from build123d import *

# Parameters (mm, degrees)
F0_R          = 25
F0_R_2        = 11.5
F1_DEPTH      = 17.5
F1_DEPTH_BACK = 17.5
F0_R_3        = 7.35
F2_DEPTH      = 6
F3_DEPTH      = 6
F4_R          = 8.4
F2_FACE_R     = 11.5
F2_FACE_R_2   = 7.35
F6_DEPTH      = 5
F3_FACE_R     = 11.5
F3_FACE_R_2   = 7.35
F7_DEPTH      = 3


with BuildPart() as f1:
    # F0 (on Front) → F1 (new body, two sides)
    with BuildSketch(Plane.XZ) as f1_sk:
        Circle(F0_R)
        Circle(F0_R_2, mode=Mode.SUBTRACT)
    extrude(amount=F1_DEPTH)
    extrude(f1_sk.sketch, amount=-F1_DEPTH_BACK)

    # F0 (on Front) → F2 (join)
    with BuildSketch(Plane.XZ):
        Circle(F0_R_2)
        Circle(F0_R_3, mode=Mode.SUBTRACT)
    extrude(amount=F2_DEPTH)

    # F0 (on Front) → F3 (join)
    with BuildSketch(Plane.XZ):
        Circle(F0_R_2)
        Circle(F0_R_3, mode=Mode.SUBTRACT)
    extrude(amount=-F3_DEPTH)

    # F4
    f4_edges = [f1.edges().sort_by_distance(p)[0] for p in [
        (-25, -17.5, 0),
        (-25, 17.5, 0),
    ]]
    fillet(f4_edges, radius=F4_R)

    # F2_face (on face) → F6 (cut)
    with BuildSketch(Plane.XZ.offset(6)):
        Circle(F2_FACE_R)
        Circle(F2_FACE_R_2, mode=Mode.SUBTRACT)
    extrude(amount=-F6_DEPTH, mode=Mode.SUBTRACT)

    # F3_face (on face) → F7 (join)
    with BuildSketch(Plane(origin=(0, 6, 0), x_dir=(1, 0, 0), z_dir=(0, 1, 0))):
        Circle(F3_FACE_R)
        Circle(F3_FACE_R_2, mode=Mode.SUBTRACT)
    extrude(amount=F7_DEPTH)


solid = f1.part
Here's how the part is built. I have some questions about the finished solid (model axes, mm). A direction names the side the tool comes from. Round coordinates to 2 decimals unless told otherwise and drop trailing zeros. Order: outer loops, then holes, each group sorted by start corner. A loop starts at its lowest first (then second) coordinate and runs counter-clockwise, first axis right, second up. Notation, with made-up numbers: M 49.25,14.25 L 88.25,14.25 A26 ccw 88.25,44.25 Z; hole C 83.5,18.25 d4. An arc over 180 degrees is marked long. Return JSON: item names as keys, results as strings. Group by question number.
1. I'm going to push flat-ended pins straight in: pin 1 Ø6 at (x, z) = (11.5, -18.5) entering from +Y; pin 2 Ø23.5 at (x, z) = (0, 0) entering from +Y; pin 3 Ø10 at (x, z) = (20, 11.5) entering from -Y; pin 4 Ø12 at (y, z) = (-3, 15) entering from +X. Where does each tip first touch, or does it pass through?
2. If we section it at B-B on z = 0: List the corners of the cut face in (x, y) for me.
3. Please list where these lines run through material, in increasing order: probe 1 along X at (y, z) = (-4, -0.5) (3 decimals); probe 2 along Z at (x, y) = (0, 0.75); probe 3 along Z at (x, y) = (0, -8).
4. If we section it at C-C on y = 1: List the corners of the cut face in (x, z) for me, then the cut area to 3 significant figures.
5. On a 3-axis mill with a long thin cutter (end or side, diameter ignored), from which of +Z, -Z, +X, -X, +Y, -Y can I reach the whole of each face in a straight line? I mean faces 5 (the face through (-4, 17.5, -11)), 6 (the face through (0, -1, -8)), 7 (the face through (-1.5, 13.2, 11.4)). Say none if no direction works.
6. If we mould it in two halves opening along Z, with no side actions, what happens to faces 1 (the face through (0, 9, 8)), 2 (the face through (-1.5, -9.1, 11.4)), 3 (the face through (23.846, -0.127, 7.509)), 4 (the face through (-4, -17.5, -11))? For each: pulls with the +Z half, pulls with the -Z half, needs draft (parallel to the pull), parting line crosses it, or undercut.
7. If we section it at A-A on x = 0: List the corners of the cut face in (y, z) for me.
8. If we section it at D-D on y = -7.5: List the corners of the cut face in (x, z) for me, then the cut area to 3 significant figures.
Reply:
{
 "1": {"pin 1": "y = 17.21", "pin 2": "y = 17.5", "pin 3": "y = -17.37", "pin 4": "x = 23.32"},
 "2": {"outline": "M -25,-9.1 A8.4 ccw -16.6,-17.5 L -11.5,-17.5 L -11.5,-1 L -7.35,-1 L -7.35,9 L -11.5,9 L -11.5,17.5 L -16.6,17.5 A8.4 ccw -25,9.1 Z; M 7.35,-1 L 11.5,-1 L 11.5,-17.5 L 16.6,-17.5 A8.4 ccw 25,-9.1 L 25,9.1 A8.4 ccw 16.6,17.5 L 11.5,17.5 L 11.5,9 L 7.35,9 Z"},
 "3": {"probe 1": "-24.995 to -11.489, 11.489 to 24.995", "probe 2": "-25 to -7.35, 7.35 to 25", "probe 3": "-25 to -11.5, 11.5 to 25"},
 "4": {"outline": "C 0,0 d50; hole C 0,0 d14.7", "area": "1,790 mm^2"},
 "5": {"face 5": "+Z, -Z, +X, -X, +Y", "face 6": "-Y", "face 7": "+Y"},
 "6": {"face 1": "undercut", "face 2": "undercut", "face 3": "parting line crosses it", "face 4": "needs draft"},
 "7": {"outline": "M -17.5,-16.6 A8.4 ccw -9.1,-25 L 9.1,-25 A8.4 ccw 17.5,-16.6 L 17.5,-11.5 L 9,-11.5 L 9,-7.35 L -1,-7.35 L -1,-11.5 L -17.5,-11.5 Z; M -17.5,11.5 L -1,11.5 L -1,7.35 L 9,7.35 L 9,11.5 L 17.5,11.5 L 17.5,16.6 A8.4 ccw 9.1,25 L -9.1,25 A8.4 ccw -17.5,16.6 Z"},
 "8": {"outline": "C 0,0 d50; hole C 0,0 d23", "area": "1,550 mm^2"}
}
